Could you check a few things on this drawing? It's one solid part, dimensions in mm from its lowest x, y, z. A direction names the side the tool comes from. Coordinates: 2 decimals unless noted, no trailing zeros. Write each loop counter-clockwise with the first axis right and the second up, starting at its lowest first coordinate (ties: lowest second). Pieces come first, ordered by that corner, then holes.
Item 1: I want a section at D-D (y = 8.25). Please give me the cut outline in (x, z).
Item 2: I'm going to push flat-ended pins straight in: P1, Ø1, axis at x = 7.5, y = 3, coming from the +Z side; P2, Ø2, axis at y = 7, z = 3.5, coming from the -X side; P3, Ø4, axis at x = 22.5, z = 13.5, coming from the +Y side; P4, Ø5, axis at y = 3.5, z = 18.5, coming from the +X side. Where does each tip first touch, or does it pass through?
Item 3: For the marked faces 1, 2, 3, 4 and 5, which set-ups out of +Z, -Z, +X, -X, +Y, -Y let a thin tool reach every point of the face, with its end or its side?
Item 4: Please list where these lines run through material, in increasing order: line 1 (X direction, y = 0.6, z = 20.5); line 2 (Z direction, x = 25, y = 0.75); line 3 (Z direction, x = 21, y = 0.65).
Item 5: I want a section at B-B (z = 7). Please give me the cut outline in (x, y).
Item 6: I want a section at A-A (x = 17). Please give me the cut outline in (y, z).
Item 7: I want a section at C-C (z = 20.5). Please give me the cut outline in (x, y), and give its area (3 significant figures).
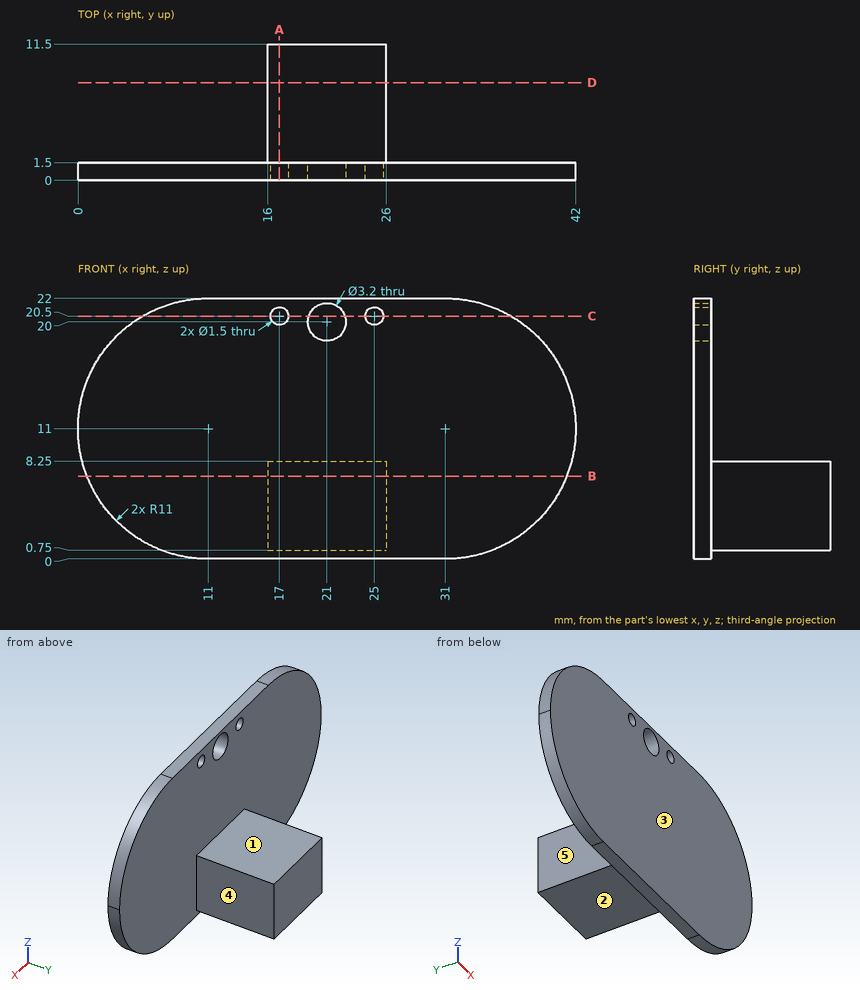
Answer:
1. outline: (16, 0.75) - (26, 0.75) - (26, 8.25) - (16, 8.25) - close
2. P1: passes through
2. P2: stops at x = 16
2. P3: stops at y = 1.5
2. P4: stops at x = 40.22
3. face 1: +Z, +X, -X, +Y
3. face 2: -Z, +X, -X, +Y
3. face 3: +Z, -Z, +X, -X, -Y
3. face 4: +Z, -Z, +X, +Y
3. face 5: +Z, -Z, -X, +Y
4. line 1: x = 5.45 to 16.25, 17.75 to 19.48, 22.52 to 24.25, 25.75 to 36.55
4. line 2: z = 0 to 19.75, 21.25 to 22
4. line 3: z = 0 to 18.4, 21.6 to 22
5. outline: (0.75, 0) - (41.25, 0) - (41.25, 1.5) - (26, 1.5) - (26, 11.5) - (16, 11.5) - (16, 1.5) - (0.75, 1.5) - close
6. outline: (0, 0) - (1.5, 0) - (1.5, 0.75) - (11.5, 0.75) - (11.5, 8.25) - (1.5, 8.25) - (1.5, 19.75) - (0, 19.75) - close; (0, 21.25) - (1.5, 21.25) - (1.5, 22) - (0, 22) - close
7. outline: (5.45, 0) - (16.25, 0) - (16.25, 1.5) - (5.45, 1.5) - close; (17.75, 0) - (19.48, 0) - (19.48, 1.5) - (17.75, 1.5) - close; (22.52, 0) - (24.25, 0) - (24.25, 1.5) - (22.52, 1.5) - close; (25.75, 0) - (36.55, 0) - (36.55, 1.5) - (25.75, 1.5) - close
7. area: 37.6 mm2
